Check sheet for the modelled part. Datum: model origin and axes. Units: mm. Face numbers are marked on the shaded views. Give positions to 0.01 mm unless a question says otherwise; leave off trailing zeros. Loops run counter-clockwise (first coordinate to the right, second up) from the corner with the lowest first, then second, coordinate; pieces in that order, holes last. Notation, with made-up numbers: (42.5, 2) - (66.5, 2) arc R27 ccw to (66.5, 28) - close; hole circle Ø7 at (41.5, 0). An arc over 180 degrees is marked (long way). Answer in a Markdown table with one row per item. Add a question column.
(1) Sectioned sample at A-A on y = 0. Enter the section's corners in (x, z), then the cut area to 3 significant figures.
(2) Thickness scan on L1, parallel to Y at x = 6.75, z = 7.5; L2, parallel to Z at x = 5.5, y = 15; L3, parallel to Z at x = 4.5, y = 0. Record the ranges inside material, lowest first.
(3) Draft check along X on the marked faces 1, 2 and 3. Enter one of: released by +X, released by -X, zero draft, split by the parting line, or undercut.
(4) Go/stop test with flat-tipped pins: P1, Ø2.5, axis at y = 16.5, z = 77, coming from the -X side; P2, Ø4, axis at y = 0, z = 17, coming from the +X side. Record where each tip stops, or that it passes through.
(5) Sectioned sample at C-C on y = 7. Enter the section's corners in (x, z).
(6) Sectioned sample at B-B on z = 75.5. Enter the section's corners in (x, y), then the cut area to 3 significant figures.
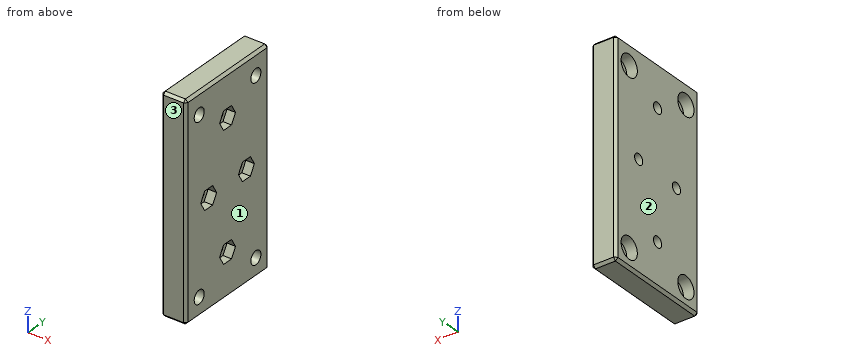
from build123d import *

# Parameters (mm, degrees)
CYLINDER014005946_R                                     = 2.65
CYLINDER014005946_DEPTH                                 = 10
CYLINDER014005947_R                                     = 2.65
CYLINDER014005947_DEPTH                                 = 10
CYLINDER014005948_R                                     = 2.65
CYLINDER014005948_DEPTH                                 = 10
CYLINDER014005949_R                                     = 4.3
CYLINDER014005949_DEPTH                                 = 4.2
CYLINDER014005950_R                                     = 4.3
CYLINDER014005950_DEPTH                                 = 4.2
CYLINDER014005951_R                                     = 4.3
CYLINDER014005951_DEPTH                                 = 4.2
CYLINDER014005952_R                                     = 4.3
CYLINDER014005952_DEPTH                                 = 4.2
PRISM015_DEPTH                                          = 3.4
CYLINDER014005953_R                                     = 2.15
CYLINDER014005953_DEPTH                                 = 16
FUSION001089102007007003008034028016007_PLACEMENT_ANGLE = 90
CYLINDER014005945_R                                     = 2.65
CYLINDER014005945_DEPTH                                 = 10
BOX021003_W                                             = 10
BOX021003_H                                             = 44
BOX021003_DEPTH                                         = 84
CHAMFER018_SIZE                                         = 1


with BuildPart() as obj1:
    # Cylinder014005946 → Cylinder014005946 (new body)
    with BuildSketch(Plane(origin=(0, 15, 7.5), x_dir=(0, 0, -1), z_dir=(1, 0, 0))):
        Circle(CYLINDER014005946_R)
    extrude(amount=CYLINDER014005946_DEPTH)


with BuildPart() as obj2:
    # Cylinder014005947 → Cylinder014005947 (new body)
    with BuildSketch(Plane(origin=(0, -15, 75.5), x_dir=(0, 0, -1), z_dir=(1, 0, 0))):
        Circle(CYLINDER014005947_R)
    extrude(amount=CYLINDER014005947_DEPTH)


with BuildPart() as obj3:
    # Cylinder014005948 → Cylinder014005948 (new body)
    with BuildSketch(Plane(origin=(0, 15, 75.5), x_dir=(0, 0, -1), z_dir=(1, 0, 0))):
        Circle(CYLINDER014005948_R)
    extrude(amount=CYLINDER014005948_DEPTH)


with BuildPart() as obj4:
    # Cylinder014005949 → Cylinder014005949 (new body)
    with BuildSketch(Plane(origin=(0, -15, 7.5), x_dir=(0, 0, -1), z_dir=(1, 0, 0))):
        Circle(CYLINDER014005949_R)
    extrude(amount=CYLINDER014005949_DEPTH)


with BuildPart() as obj5:
    # Cylinder014005950 → Cylinder014005950 (new body)
    with BuildSketch(Plane(origin=(0, 15, 7.5), x_dir=(0, 0, -1), z_dir=(1, 0, 0))):
        Circle(CYLINDER014005950_R)
    extrude(amount=CYLINDER014005950_DEPTH)


with BuildPart() as obj6:
    # Cylinder014005951 → Cylinder014005951 (new body)
    with BuildSketch(Plane(origin=(0, -15, 75.5), x_dir=(0, 0, -1), z_dir=(1, 0, 0))):
        Circle(CYLINDER014005951_R)
    extrude(amount=CYLINDER014005951_DEPTH)


with BuildPart() as obj7:
    # Cylinder014005952 → Cylinder014005952 (new body)
    with BuildSketch(Plane(origin=(0, 15, 75.5), x_dir=(0, 0, -1), z_dir=(1, 0, 0))):
        Circle(CYLINDER014005952_R)
    extrude(amount=CYLINDER014005952_DEPTH)


with BuildPart() as m4x007:
    # prism015 → prism015 (new body)
    with BuildSketch(Plane(origin=(0, 0, 0), x_dir=(0, 1, 0), z_dir=(0, 0, 1))):
        Polygon((4.21, 0), (2.105, 3.645967), (-2.105, 3.645967), (-4.21, 0), (-2.105, -3.645967), (2.105, -3.645967), align=None)
    extrude(amount=PRISM015_DEPTH)


with BuildPart() as m4nut025:
    # Cylinder014005953 → Cylinder014005953 (new body)
    with BuildSketch(Plane.XY):
        Circle(CYLINDER014005953_R)
    extrude(amount=CYLINDER014005953_DEPTH)

    # Fusion001089102007007003008034028016007: union M4X007
    add(m4x007.part)


with BuildPart() as m4nut025_1:
    # Fusion001089102007007003008034028016007 placement: moved
    add(m4nut025.part.moved(Location((10, 0, 42))).rotate(Axis((10, 0, 42), (0, -1, 0)), FUSION001089102007007003008034028016007_PLACEMENT_ANGLE))


with BuildPart() as m4nut026:
    # Fusion001089102007007003008034028016007001 base: copy of M4nut025
    add(m4nut025_1.part)


with BuildPart() as m4nut026_1:
    # Fusion001089102007007003008034028016007001 placement: moved
    add(m4nut026.part.moved(Location((0, 10, 1))))


with BuildPart() as m4nut027:
    # Fusion001089102007007003008034028016007002 base: copy of M4nut025
    add(m4nut025_1.part)


with BuildPart() as m4nut027_1:
    # Fusion001089102007007003008034028016007002 placement: moved
    add(m4nut027.part.moved(Location((0, -10, 0))))


with BuildPart() as m4nut029:
    # Fusion001089102007007003008034028016007004 base: copy of M4nut025
    add(m4nut025_1.part)


with BuildPart() as m4nut029_1:
    # Fusion001089102007007003008034028016007004 placement: moved
    add(m4nut029.part.moved(Location((0, 0, -25))))


with BuildPart() as m4nut028:
    # Fusion001089102007007003008034028016007003 base: copy of M4nut025
    add(m4nut025_1.part)


with BuildPart() as m4nut028_1:
    # Fusion001089102007007003008034028016007003 placement: moved
    add(m4nut028.part.moved(Location((0, 0, 25))))


with BuildPart() as fusion001089102007007003008034028016006:
    # Cylinder014005945 → Cylinder014005945 (new body)
    with BuildSketch(Plane(origin=(0, -15, 7.5), x_dir=(0, 0, -1), z_dir=(1, 0, 0))):
        Circle(CYLINDER014005945_R)
    extrude(amount=CYLINDER014005945_DEPTH)

    # Fusion001089102007007003008034028016006: union obj1, obj2, obj3, obj4, obj5, obj6, obj7, M4nut026, M4nut027, M4nut029, M4nut028
    add(obj1.part)
    add(obj2.part)
    add(obj3.part)
    add(obj4.part)
    add(obj5.part)
    add(obj6.part)
    add(obj7.part)
    add(m4nut026_1.part)
    add(m4nut027_1.part)
    add(m4nut029_1.part)
    add(m4nut028_1.part)


with BuildPart() as chamfer018:
    # Box021003 → Box021003 (new body)
    with BuildSketch(Plane(origin=(0, -22, 0), x_dir=(1, 0, 0), z_dir=(0, 0, 1))):
        with Locations((5, 22)):
            Rectangle(BOX021003_W, BOX021003_H)
    extrude(amount=BOX021003_DEPTH)

    # Cut009003003009003003003007003002002: cut Fusion001089102007007003008034028016006
    add(fusion001089102007007003008034028016006.part, mode=Mode.SUBTRACT)

    # Chamfer018
    chamfer018_edges = [chamfer018.edges().sort_by_distance(p)[0] for p in [
        (0, -22, 42),
        (0, 0, 84),
        (0, 0, 0),
        (0, 22, 42),
        (5, -22, 0),
        (10, -22, 42),
        (5, -22, 84),
        (5, 22, 84),
        (10, 0, 84),
        (5, 22, 0),
        (10, 0, 0),
        (10, 22, 42),
    ]]
    chamfer(chamfer018_edges, length=CHAMFER018_SIZE)


solid = chamfer018.part
Reply:
| question | item | result |
|---|---|---|
| 1 | outline | (0, 1) - (1, 0) - (9, 0) - (10, 1) - (10, 13.35) - (6.6, 13.35) - (6.6, 14.85) - (0, 14.85) - close; (0, 19.15) - (6.6, 19.15) - (6.6, 20.65) - (10, 20.65) - (10, 63.35) - (6.6, 63.35) - (6.6, 64.85) - (0, 64.85) - close; (0, 69.15) - (6.6, 69.15) - (6.6, 70.65) - (10, 70.65) - (10, 83) - (9, 84) - (1, 84) - (0, 83) - close |
| 1 | area | 732 mm^2 |
| 2 | L1 | -22 to -17.65, -12.35 to 12.35, 17.65 to 22 |
| 2 | L2 | 0 to 4.85, 10.15 to 72.85, 78.15 to 84 |
| 2 | L3 | 0 to 14.85, 19.15 to 64.85, 69.15 to 84 |
| 3 | face 1 | released by +X |
| 3 | face 2 | released by -X |
| 3 | face 3 | zero draft |
| 4 | P1 | x = 4.2 |
| 4 | P2 | through |
| 5 | outline | (0, 1) - (1, 0) - (9, 0) - (10, 1) - (10, 40.9) - (6.6, 40.9) - (6.6, 45.1) - (10, 45.1) - (10, 83) - (9, 84) - (1, 84) - (0, 83) - close |
| 6 | outline | (0, -21) - (1, -22) - (9, -22) - (10, -21) - (10, -17.65) - (4.2, -17.65) - (4.2, -19.3) - (0, -19.3) - close; (0, -10.7) - (4.2, -10.7) - (4.2, -12.35) - (10, -12.35) - (10, 12.35) - (4.2, 12.35) - (4.2, 10.7) - (0, 10.7) - close; (0, 19.3) - (4.2, 19.3) - (4.2, 17.65) - (10, 17.65) - (10, 21) - (9, 22) - (1, 22) - (0, 21) - close |
| 6 | area | 304 mm^2 |
